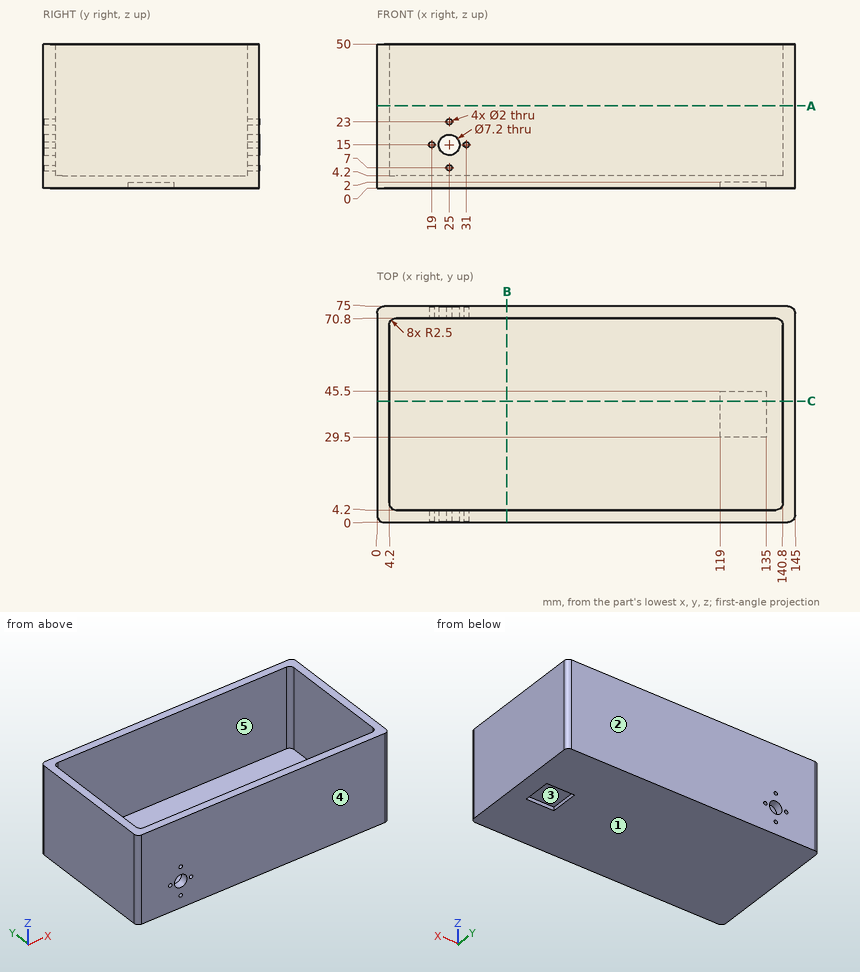
Here's the drawing with two shaded views (mm, measured from the low corner). I have some questions. A direction names the side the tool comes from. Coordinates: 2 decimals unless noted, no trailing zeros. Write each loop counter-clockwise with the first axis right and the second up, starting at its lowest first coordinate (ties: lowest second). Pieces come first, ordered by that corner, then holes. Notation, with made-up numbers: (39, 30) -> (64, 30) arc R19 cw to (64, 43) -> close; hole circle Ø3 at (-28, 34.5). An arc over 180 degrees is marked (long way). Use a Markdown table: item, result. Add a question column.
(1) If we section it at B-B, the plane x = 45: Write out the boundary of the cut face in (y, z).
(2) For the marked faces 4 and 5, which set-ups out of +Z, -Z, +X, -X, +Y, -Y let a thin tool reach every point of the face, with its end or its side?
(3) If we section it at A-A, the plane z = 28.5: Write out the boundary of the cut face in (x, y).
(4) I'm going to push flat-ended pins straight in: P1, Ø8, axis at x = 59.5, y = 19, coming from the +Z side; P2, Ø3, axis at x = 129, y = 32, coming from the -Z side. Where does each tip first touch, or does it pass through?
(5) We'd pull the mould along Y, two halves only. Please class the marked faces 1, 2 and 3: +Y half, -Y half, draft (parallel to the pull), parting line (faces both ways), or undercut.
(6) If we section it at C-C, the plane y = 42: Write out the boundary of the cut face in (x, z), and give its area (3 significant figures).
(7) Please list where these lines run through material, in increasing order: line 1 (Z direction, x = 25, y = 1.7); line 2 (Y direction, x = 78.5, z = 33); line 3 (X direction, y = 59, z = 48.5).
Outcome:
| question | item | result |
|---|---|---|
| 1 | outline | (0, 0) -> (75, 0) -> (75, 50) -> (70.8, 50) -> (70.8, 4.2) -> (4.2, 4.2) -> (4.2, 50) -> (0, 50) -> close |
| 2 | face 4 | +Z, -Z, +X, -X, -Y |
| 2 | face 5 | +Z |
| 3 | outline | (0, 2.5) arc R2.5 ccw to (2.5, 0) -> (142.5, 0) arc R2.5 ccw to (145, 2.5) -> (145, 72.5) arc R2.5 ccw to (142.5, 75) -> (2.5, 75) arc R2.5 ccw to (0, 72.5) -> close; hole (4.2, 6.7) arc R2.5 ccw to (6.7, 4.2) -> (138.3, 4.2) arc R2.5 ccw to (140.8, 6.7) -> (140.8, 68.3) arc R2.5 ccw to (138.3, 70.8) -> (6.7, 70.8) arc R2.5 ccw to (4.2, 68.3) -> close |
| 4 | P1 | stops at z = 4.2 |
| 4 | P2 | stops at z = 2 |
| 5 | face 1 | draft |
| 5 | face 2 | +Y half |
| 5 | face 3 | undercut |
| 6 | outline | (0, 0) -> (119, 0) -> (119, 2) -> (135, 2) -> (135, 0) -> (145, 0) -> (145, 50) -> (140.8, 50) -> (140.8, 4.2) -> (4.2, 4.2) -> (4.2, 50) -> (0, 50) -> close |
| 6 | area | 962 mm^2 |
| 7 | line 1 | z = 0 to 6, 8 to 11.4, 18.6 to 22, 24 to 50 |
| 7 | line 2 | y = 0 to 4.2, 70.8 to 75 |
| 7 | line 3 | x = 0 to 4.2, 140.8 to 145 |
